Geometry check sheet. Reference: the model listing, model coordinates, mm. Face numbers are marked on the shaded views. Coordinates: 2 decimals unless noted, no trailing zeros. Loops run counter-clockwise (first coordinate to the right, second up) from the corner with the lowest first, then second, coordinate; pieces in that order, holes last. Notation, with made-up numbers: (57.5, 52) - (106.5, 52) arc R32 ccw to (106.5, 84) - close; hole circle Ø8 at (42, -38). An arc over 180 degrees is marked (long way). One line per item, written item: value.
from build123d import *

# Parameters (mm, degrees)
BOSS_EXTRUDE1_DEPTH  = 76.2
CUT_EXTRUDE1_START   = -27.572978
CUT_EXTRUDE1_DEPTH   = 55.145956
M3_CLEARANCE_HOLE1_D = 3.4
CUT_EXTRUDE2_REACH   = 149.802
SKETCH10_R           = 19.05


with BuildPart() as part:
    # Sketch1 → Boss-Extrude1 (new body)
    with BuildSketch(Plane.XY):
        Polygon((27.572977546, -123.606903324), (27.572977546, -70.715393761), (0, -4.148337413), (-27.572977546, -70.715393761), (-27.572977546, -123.606903324), align=None)
    extrude(amount=BOSS_EXTRUDE1_DEPTH)

    # Sketch2 → Cut-Extrude1 (cut)
    with BuildSketch(Plane(origin=(0, 0, 0), x_dir=(0, 0, -1), z_dir=(1, 0, 0)).offset(CUT_EXTRUDE1_START)):
        with BuildLine():
            Line((-76.2, -123.606903324), (0, -123.606903324))
            ThreePointArc((0, -123.606903324), (-26.454151539, -62.84107661), (-76.2, -19.05))
            Line((-76.2, -19.05), (-76.2, -70.715393761))
            Line((-76.2, -70.715393761), (-76.2, -123.606903324))
        make_face()
    extrude(amount=CUT_EXTRUDE1_DEPTH, mode=Mode.SUBTRACT)

    # M3 Clearance Hole1 (through all)
    with Locations(Plane(origin=(0, 0, 0), x_dir=(-1, 0, 0), z_dir=(0, 0, -1))):
        with Locations((-15.875, -81.009177721), (15.875, -81.009177721), (0, -38.1)):
            Hole(M3_CLEARANCE_HOLE1_D / 2)

    # Sketch10 → Cut-Extrude2 (cut, up to next)
    with BuildSketch(Plane(origin=(0, 0, 0), x_dir=(-1, 0, 0), z_dir=(0, 0, -1)), mode=Mode.PRIVATE) as cut_extrude2_sk1:
        Circle(SKETCH10_R)
    cut_extrude2_tool1 = extrude(cut_extrude2_sk1.sketch, amount=-CUT_EXTRUDE2_REACH, mode=Mode.PRIVATE) & part.part
    add(cut_extrude2_tool1.solids().sort_by_distance((0, 0, 0))[0], mode=Mode.SUBTRACT)


solid = part.part
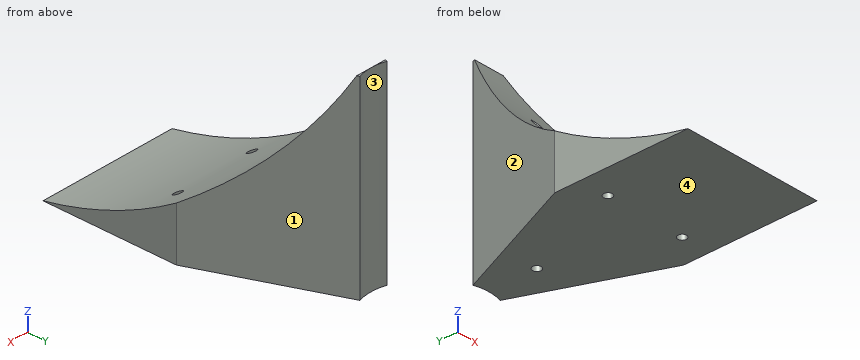
(1) Go/stop test with flat-tipped pins: pin 1 Ø2 at (x, z) = (1, 17) entering from -Y; pin 2 Ø4 at (x, y) = (-7.5, -62.5) entering from -Z; pin 3 Ø4 at (x, z) = (-22, 12) entering from -Y; pin 4 Ø3 at (x, z) = (-4, 19.5) entering from +Y. Record where each tip stops, or that it passes through.
Reply:
pin 1: y = -79.3
pin 2: z = 0
pin 3: y = -91.5
pin 4: y = -18.24
(2) Cross-section at D-D on y = -92.5. Record the cut outline in (x, z), and give its area (3 significant figures).
Reply:
outline: (-27.57, 0) - (27.57, 0) - (27.57, 9.57) - (-27.57, 9.57) - close
area: 528 mm2
(3) Release check for a two-part mould opening along X. For the marked faces 1, 2, 3 and 4 record: pulls with the +X half, pulls with the -X half, needs draft (parallel to the pull), parting line crosses it, or undercut.
Reply:
face 1: pulls with the +X half
face 2: pulls with the -X half
face 3: undercut
face 4: needs draft
(4) Material ranges on probe 1 along Y at (x, z) = (0, 20); probe 2 along Y at (x, z) = (0, 11.5); probe 3 along Z at (x, y) = (7.5, -23.5), recorded low to high. Write a range as from..to.
Reply:
probe 1: -72.44..-39.8, -36.4..-19.05
probe 2: -88.18..-39.8, -36.4..-19.05
probe 3: 0..68.63
(5) Cross-section at C-C on x = -23.5. Record the cut outline in (y, z), and give its area (3 significant figures).
Reply:
outline: (-123.61, 0) - (-60.88, 0) - (-60.88, 27.91) arc R152.4 cw to start
area: 695 mm2
(6) Cross-section at B-B on z = 35.5. Record the cut outline in (x, y).
Reply:
outline: (-19.65, -51.59) - (19.65, -51.59) - (5.8, -18.15) arc R19.05 cw to (-5.8, -18.15) - close; hole circle Ø3.4 at (0, -38.1)
(7) Cross-section at A-A on y = -38.1. Record the cut outline in (x, z).
Reply:
outline: (-14.06, 0) - (-1.7, 0) - (-1.7, 49.04) - (-14.06, 49.04) - close; (1.7, 0) - (14.06, 0) - (14.06, 49.04) - (1.7, 49.04) - close
